```python
from build123d import *

# Parameters (mm, degrees)
EXTRUDE_THIN1_DEPTH   = 30
EXTRUDE_THIN1_2_DEPTH = 30
BOSS_EXTRUDE1_START   = -1
BOSS_EXTRUDE1_DEPTH   = 1
BOSS_EXTRUDE2_DEPTH   = 1
FILLET1_R             = 10
FILLET2_R             = 5


with BuildPart() as part:
    # Sketch1 → Extrude-Thin1 (new body)
    with BuildSketch(Plane.XY):
        with BuildLine():
            Line((0, 0), (0, -9.941978892))
            Line((0, -9.941978892), (0, -13.23222107))
            ThreePointArc((0, -13.23222107), (4.393398282, -23.838822788), (15, -28.23222107))
            Line((15, -28.23222107), (40.06481759, -28.23222107))
            Line((40.06481759, -28.23222107), (40.06481759, -27.23222107))
            Line((40.06481759, -27.23222107), (15, -27.23222107))
            ThreePointArc((15, -27.23222107), (5.100505063, -23.131716006), (1, -13.23222107))
            Line((1, -13.23222107), (1, -9.941978892))
            Line((1, -9.941978892), (1, 0))
            Line((1, 0), (0, 0))
        make_face()
    extrude(amount=EXTRUDE_THIN1_DEPTH)



with BuildPart() as body_2:
    # Sketch1 → Extrude-Thin1 2 (new body)
    with BuildSketch(Plane.XY):
        with BuildLine():
            Line((22, 0), (22, -9.941978892))
            Line((22, -9.941978892), (22, -12.525749024))
            ThreePointArc((22, -12.525749024), (24.928932188, -19.596816836), (32, -22.525749024))
            Line((32, -22.525749024), (40.06481759, -22.525749024))
            Line((40.06481759, -22.525749024), (44.344767003, -26.773486601))
            Line((44.344767003, -26.773486601), (45.049197787, -26.063713912))
            Line((45.049197787, -26.063713912), (40.476820184, -21.525749024))
            Line((40.476820184, -21.525749024), (32, -21.525749024))
            ThreePointArc((32, -21.525749024), (25.636038969, -18.889710055), (23, -12.525749024))
            Line((23, -12.525749024), (23, -9.941978892))
            Line((23, -9.941978892), (23, 0))
            Line((23, 0), (22, 0))
        make_face()
    extrude(amount=EXTRUDE_THIN1_2_DEPTH)


with BuildPart() as part_1:
    add(part.part)

    add(body_2.part)  # Boss-Extrude1 merges body 2
    # Sketch2 → Boss-Extrude1 (add)
    with BuildSketch(Plane.XY.offset(30).offset(BOSS_EXTRUDE1_START)):
        with BuildLine():
            Line((40.476820184, -21.525749024), (32, -21.525749024))
            ThreePointArc((32, -21.525749024), (25.636038969, -18.889710055), (23, -12.525749024))
            Line((23, -12.525749024), (23, 0))
            Line((23, 0), (22, 0))
            Line((22, 0), (1, 0))
            Line((1, 0), (0, 0))
            Line((0, 0), (0, -13.23222107))
            ThreePointArc((0, -13.23222107), (4.393398282, -23.838822788), (15, -28.23222107))
            Line((15, -28.23222107), (40.06481759, -28.23222107))
            Line((40.06481759, -28.23222107), (44.344767003, -26.773486601))
            Line((44.344767003, -26.773486601), (45.049197787, -26.063713912))
            Line((45.049197787, -26.063713912), (40.476820184, -21.525749024))
        make_face()
    extrude(amount=BOSS_EXTRUDE1_DEPTH)

    # Sketch3 → Boss-Extrude2 (add)
    with BuildSketch(Plane(origin=(0, 0, 0), x_dir=(-1, 0, 0), z_dir=(0, 0, -1))):
        with BuildLine():
            Line((-44.344767003, -26.773486601), (-40.06481759, -28.23222107))
            Line((-40.06481759, -28.23222107), (-15, -28.23222107))
            ThreePointArc((-15, -28.23222107), (-4.393398282, -23.838822788), (0, -13.23222107))
            Line((0, -13.23222107), (0, 0))
            Line((0, 0), (-1, 0))
            Line((-1, 0), (-22, 0))
            Line((-22, 0), (-23, 0))
            Line((-23, 0), (-23, -12.525749024))
            ThreePointArc((-23, -12.525749024), (-25.636038969, -18.889710055), (-32, -21.525749024))
            Line((-32, -21.525749024), (-40.476820184, -21.525749024))
            Line((-40.476820184, -21.525749024), (-45.049197787, -26.063713912))
            Line((-45.049197787, -26.063713912), (-44.344767003, -26.773486601))
        make_face()
    extrude(amount=-BOSS_EXTRUDE2_DEPTH)

    # Fillet1
    fillet1_edges = [part_1.edges().sort_by_distance(p)[0] for p in [
        (40.476820184, -21.525749024, 15),
        (40.06481759, -22.525749024, 15),
    ]]
    fillet(fillet1_edges, radius=FILLET1_R)

    # Fillet2
    # the kernel refuses this fillet: 5 mm, written as the material it takes off along each edge
    with BuildSketch(Plane(origin=(40.06481759, -27.23222107, 1), x_dir=(0, -1, 0), z_dir=(0, 0, 1))) as fillet2_piece_1:
        with BuildLine():
            CenterArc((5, -3), FILLET2_R, 143.130102354, 36.869897646)
            Line((0, -3), (0, 0))
            Line((0, 0), (1, 0))
        make_face()
    extrude(amount=28, mode=Mode.SUBTRACT)


solid = part_1.part
```
Geometry: final body of the model. Coordinates: model frame, mm. A direction names the side the tool comes from. Round coordinates to 2 decimals unless told otherwise and drop trailing zeros. Order: outer loops, then holes, each group sorted by start corner. A loop starts at its lowest first (then second) coordinate and runs counter-clockwise, first axis right, second up. Notation, with made-up numbers: M 72,26.5 L 104,26.5 A24 ccw 104,61.5 Z; hole C 37,-12.75 d1. An arc over 180 degrees is marked long. One line per item, written item: value.
(1) Cut plane C-C (x = 27). Return the cut outline in (y, z), and give its area (3 significant figures).
Result sheet:
outline: M -28.23,0 L -20.01,0 L -20.01,30 L -28.23,30 Z; hole M -27.23,1 L -21.19,1 L -21.19,29 L -27.23,29 Z
area: 77.4 mm2
(2) Line query: probe 1 along X at (y, z) = (-10.5, 11); probe 2 along Y at (x, z) = (32, 21); probe 3 along Z at (x, y) = (14, -5.5). Output: solid intervals per line, ascending. Write a range as [from, to].
Result sheet:
probe 1: [0, 1], [22, 23]
probe 2: [-28.23, -27.23], [-22.53, -21.53]
probe 3: [0, 1], [29, 30]
(3) Cut plane B-B (y = -11). Return the cut outline in (x, z).
Result sheet:
outline: M 0,0 L 23,0 L 23,30 L 0,30 Z; hole M 1,1 L 22,1 L 22,29 L 1,29 Z
(4) Reachability of faces 4 (the flat face through (23, -6, 15)), 5 (the flat face through (26, -27.232, 15)), 6 (the cylindrical face through (39.704, -23.259, 15.196)), 7 (the cylindrical face through (5.21, -23.24, 14.8)) from +Z, -Z, +X, -X, +Y, -Y: full face, straight path, thin tool, end or side. Return the list, or none.
Result sheet:
face 4: +Z, -Z, +X, +Y
face 5: +X
face 6: none
face 7: +Y
(5) Cut plane D-D (x = 12.5). Return the cut outline in (y, z), and give its area (3 significant figures).
Result sheet:
outline: M -28.02,0 L 0,0 L 0,1 L -27.01,1 L -27.01,29 L 0,29 L 0,30 L -28.02,30 Z
area: 84.5 mm2
(6) Pin query (flat end, axial travel): P1, Ø14, axis at x = 30.5, y = -12, coming from the -Z side; P2, Ø1.5, axis at x = 7.5, z = 23.5, coming from the +Y side; P3, Ø5, axis at y = -20.5, z = 15, coming from the +X side; P4, Ø1, axis at y = -23, z = 9, coming from the -X side. Return the tip coordinate at first contact, or that it passes through.
Result sheet:
P1: through
P2: y = -24.54
P3: x = 41.58
P4: x = 3.21
(7) Pull-direction query (Z, two-part tool) for faces 1 (the flat face through (17, -14, 30)), 2 (the flat face through (1, -7, 15)), 3 (the flat face through (27, -28.232, 15)); classes: pulls with the +Z half, pulls with the -Z half, needs draft (parallel to the pull), parting line crosses it, or undercut.
Result sheet:
face 1: pulls with the +Z half
face 2: undercut
face 3: needs draft
(8) Cut plane A-A (z = 25.25). Return the cut outline in (x, y), and give its area (3 significant figures).
Result sheet:
outline: M 0,-13.23 A15 ccw 15,-28.23 L 40.06,-28.23 A5 ccw 37.06,-27.23 L 15,-27.23 A14 cw 1,-13.23 L 1,0 L 0,0 Z; M 22,-12.53 A10 ccw 32,-22.53 L 35.94,-22.53 A10 cw 42.99,-25.43 L 44.34,-26.77 L 45.05,-26.06 L 43.4,-24.43 A10 ccw 36.36,-21.53 L 32,-21.53 A9 cw 23,-12.53 L 23,0 L 22,0 Z
area: 102 mm2
